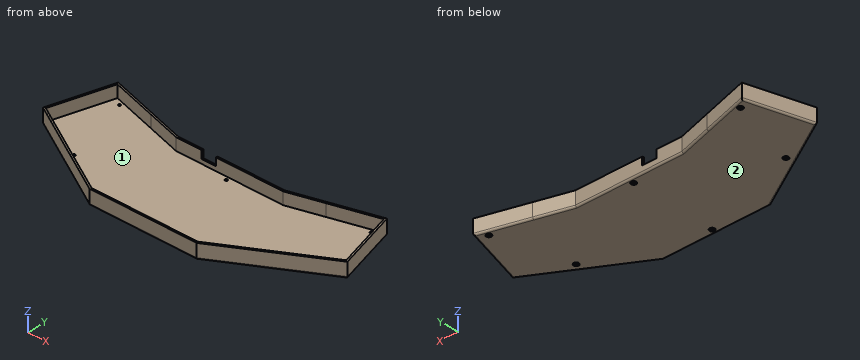
```python
from build123d import *

# Parameters (mm, degrees)
BOSS_EXTRU_1_DEPTH      = 14
BOSS_EXTRU_2_DEPTH      = 3
CONG_1_R                = 2
ENL_V_START             = 5
ENL_V_MAT_EXTRU_1_DEPTH = 10
ESQUISSE7_R             = 1.5
ENL_V_MAT_EXTRU_2_DEPTH = 10
ESQUISSE8_R             = 3
ENL_V_MAT_EXTRU_3_DEPTH = 2


with BuildPart() as part:
    # Esquisse1 → Boss.-Extru.1 (new body)
    with BuildSketch(Plane.XY):
        Polygon((229.15721289, -14.84723942), (106.433306853, -14.84723942), (67.372523259, -3.649091023), (12.961214213, 11.953100779), (-7.58450021, -59.698320459), (106.05278448, -124.898736851), (229.537735263, -124.898736851), (343.175019953, -59.698320459), (322.62930553, 11.953100779), (268.217996484, -3.649091023), align=None)
        Polygon((229.438237844, -16.84723942), (106.152281899, -16.84723942), (66.821302011, -5.571629745), (14.332462893, 9.479302675), (-5.230075099, -58.743374877), (106.585792597, -122.898736851), (229.004727146, -122.898736851), (340.820594842, -58.743374877), (321.25805685, 9.479302675), (268.769217732, -5.571629745), align=None, mode=Mode.SUBTRACT)
    extrude(amount=BOSS_EXTRU_1_DEPTH)

    # Esquisse2 → Boss.-Extru.2 (add)
    with BuildSketch(Plane(origin=(0, 0, 0), x_dir=(-1, 0, 0), z_dir=(0, 0, -1))):
        Polygon((-229.15721289, -14.84723942), (-268.217996484, -3.649091023), (-322.62930553, 11.953100779), (-343.175019953, -59.698320459), (-229.537735263, -124.898736851), (-106.05278448, -124.898736851), (7.58450021, -59.698320459), (-12.961214213, 11.953100779), (-67.372523259, -3.649091023), (-106.433306853, -14.84723942), align=None)
    extrude(amount=BOSS_EXTRU_2_DEPTH)

    # Congé1
    cong_1_edges = [part.edges().sort_by_distance(p)[0] for p in [
        (167.795259872, -14.84723942, -3),
        (248.687604687, -9.248165222, -3),
        (295.423651007, 4.152004878, -3),
        (332.902162742, -23.87260984, -3),
        (286.356377608, -92.298528655, -3),
        (167.795259872, -124.898736851, -3),
        (49.234142135, -92.298528655, -3),
        (2.688357001, -23.87260984, -3),
        (40.166868736, 4.152004878, -3),
        (86.902915056, -9.248165222, -3),
    ]]
    fillet(cong_1_edges, radius=CONG_1_R)

    # Esquisse3 → Enlèv. mat.-Extru.1 (cut)
    with BuildSketch(Plane.XY.offset(ENL_V_START)):
        Polygon((142.206494045, 6.988548589), (157.586708491, 2.578446141), (132.665816954, -84.333062282), (117.285602508, -79.922959834), align=None)
    extrude(amount=ENL_V_MAT_EXTRU_1_DEPTH, mode=Mode.SUBTRACT)

    # Esquisse7 → Enlèv. mat.-Extru.2 (cut)
    with BuildSketch(Plane.XY):
        with Locations((312.747989314, 2.877882334)):
            Circle(ESQUISSE7_R)
        with Locations((167.795259872, -20.84723942)):
            Circle(ESQUISSE7_R)
        with Locations(Location((22.842530429, 2.877882334, 0), (0, 0, 180))):
            Circle(ESQUISSE7_R)
        with Locations(Location((167.795259872, -118.898736851, 0), (0, 0, 180))):
            Circle(ESQUISSE7_R)
        with Locations((46.946880967, -80.077290604)):
            Circle(ESQUISSE7_R)
        with Locations(Location((288.643638776, -80.077290604, 0), (0, 0, 180))):
            Circle(ESQUISSE7_R)
    extrude(amount=-ENL_V_MAT_EXTRU_2_DEPTH, mode=Mode.SUBTRACT)

    # Esquisse8 → Enlèv. mat.-Extru.3 (cut)
    with BuildSketch(Plane(origin=(0, 0, -3), x_dir=(-1, 0, 0), z_dir=(0, 0, -1))):
        with Locations((-22.842530429, 2.877882334)):
            Circle(ESQUISSE8_R)
        with Locations((-46.946880967, -80.077290604)):
            Circle(ESQUISSE8_R)
        with Locations((-167.795259872, -118.898736851)):
            Circle(ESQUISSE8_R)
        with Locations((-167.795259872, -20.84723942)):
            Circle(ESQUISSE8_R)
        with Locations((-288.643638776, -80.077290604)):
            Circle(ESQUISSE8_R)
        with Locations((-312.747989314, 2.877882334)):
            Circle(ESQUISSE8_R)
    extrude(amount=-ENL_V_MAT_EXTRU_3_DEPTH, mode=Mode.SUBTRACT)


solid = part.part
```
Geometry: final body of the model. Coordinates: model frame, mm. Face numbers are marked on the shaded views. Round coordinates to 2 decimals unless told otherwise and drop trailing zeros. Order: outer loops, then holes, each group sorted by start corner. A loop starts at its lowest first (then second) coordinate and runs counter-clockwise, first axis right, second up. Notation, with made-up numbers: (23.25, -37) -> (27.25, -37) arc R10 ccw to (27.25, -25) -> close; hole circle Ø1 at (35, -15). An arc over 180 degrees is marked (long way). Use one line per item in the form item = value.
(1) First-contact query: pin 1 Ø5 at (y, z) = (-96, 4.5) entering from +X; pin 2 Ø1.8 at (x, y) = (166.5, -120) entering from -Z; pin 3 Ø5 at (y, z) = (-62.5, 1) entering from +X. Flat tips, straight axial feed; report the tip coordinate or a pass-through.
Results list:
pin_1 = 284.26
pin_2 = -1
pin_3 = 342.65
(2) Draft query along Y for the marked faces 1 and 2. Return one class per face: pulls with the +Y half, pulls with the -Y half, needs draft (parallel to the pull), parting line crosses it, or undercut.
Results list:
face_1 = undercut
face_2 = needs draft
(3) Section B-B on x = 199. Return loops of the section in (y, z).
Results list:
outline = (-124.9, -1) arc R2 ccw to (-122.9, -3) -> (-16.85, -3) arc R2 ccw to (-14.85, -1) -> (-14.85, 14) -> (-16.85, 14) -> (-16.85, 0) -> (-122.9, 0) -> (-122.9, 14) -> (-124.9, 14) -> close
(4) Ray query, probe 1 along Y at (x, z) = (226, 2); probe 2 along Z at (x, y) = (150, -43); probe 3 along Y at (x, z) = (298.5, 11.5). Return the intervals inside material, ascending. Write a range as [from, to].
Results list:
probe_1 = [-124.9, -122.9], [-16.85, -14.85]
probe_2 = [-3, 0]
probe_3 = [-85.33, -83.03], [2.95, 5.03]
(5) Section A-A on z = 10. Return loops of the section in (x, y), and give its area (3 significant figures).
Results list:
outline = (-7.58, -59.7) -> (106.05, -124.9) -> (229.54, -124.9) -> (343.18, -59.7) -> (322.63, 11.95) -> (268.22, -3.65) -> (229.16, -14.85) -> (152.59, -14.85) -> (152.02, -16.85) -> (229.44, -16.85) -> (268.77, -5.57) -> (321.26, 9.48) -> (340.82, -58.74) -> (229, -122.9) -> (106.59, -122.9) -> (-5.23, -58.74) -> (14.33, 9.48) -> (66.82, -5.57) -> (106.15, -16.85) -> (135.37, -16.85) -> (135.95, -14.85) -> (106.43, -14.85) -> (67.37, -3.65) -> (12.96, 11.95) -> close
area = 1,660 mm^2
